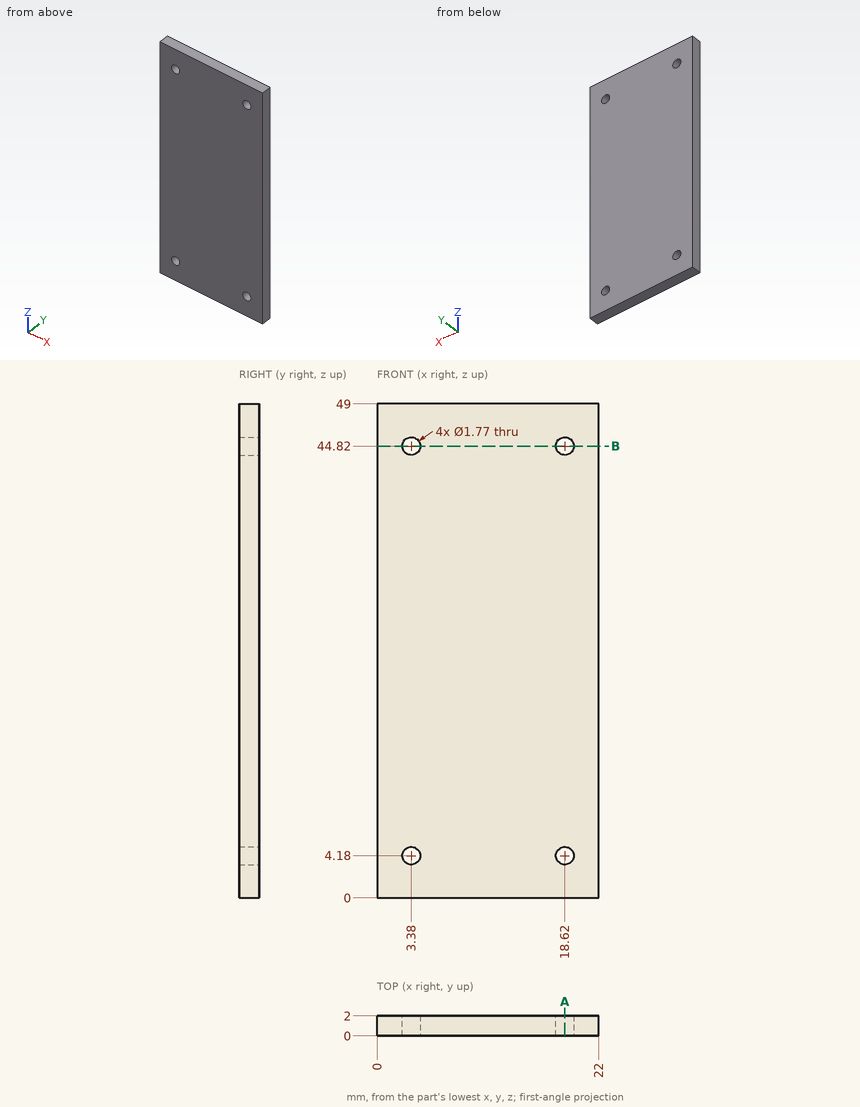
Geometry: see drawing. Coordinates: mm, zero at the bounding-box minimum. Coordinates: 2 decimals unless noted, no trailing zeros. Loops run counter-clockwise (first coordinate to the right, second up) from the corner with the lowest first, then second, coordinate; pieces in that order, holes last. Notation, with made-up numbers: (18.25, -8) -> (54.25, -8) arc R22 ccw to (54.25, 20) -> close; hole circle Ø7 at (9, 44). An arc over 180 degrees is marked (long way). Write item = value, one per line. Start each with the question number.
Item 1: Material intervals for line 1 (X direction, y = 0.7, z = 44.82) (3 decimals); line 2 (Z direction, x = 3.38, y = 1.1) (3 decimals); line 3 (Z direction, x = 19, y = 1.35), sorted ascending.
Item 2: Cut plane B-B, the plane z = 44.82. Return loops of the section in (x, y) (3 decimals), plus the area to 3 significant figures.
Item 3: Cut plane A-A, the plane x = 18.62. Return loops of the section in (y, z) (3 decimals), plus the area to 3 significant figures.
Item 4: First-contact query: P1, Ø2, axis at x = 14.5, z = 36.5, coming from the -Y side; P2, Ø1.1, axis at x = 3.38, z = 4.18, coming from the -Y side. Flat tips, straight axial feed; report the tip coordinate or a pass-through.
Ans:
q1.line_1 = 0 to 2.495, 4.265 to 17.735, 19.505 to 22
q1.line_2 = 0 to 3.295, 5.065 to 43.935, 45.705 to 49
q1.line_3 = 0 to 3.38, 4.98 to 44.02, 45.62 to 49
q2.outline = (0, 0) -> (2.495, 0) -> (2.495, 2) -> (0, 2) -> close; (4.265, 0) -> (17.735, 0) -> (17.735, 2) -> (4.265, 2) -> close; (19.505, 0) -> (22, 0) -> (22, 2) -> (19.505, 2) -> close
q2.area = 36.9 mm²
q3.outline = (0, 0) -> (2, 0) -> (2, 3.295) -> (0, 3.295) -> close; (0, 5.065) -> (2, 5.065) -> (2, 43.935) -> (0, 43.935) -> close; (0, 45.705) -> (2, 45.705) -> (2, 49) -> (0, 49) -> close
q3.area = 90.9 mm²
q4.P1 = 0
q4.P2 = through
